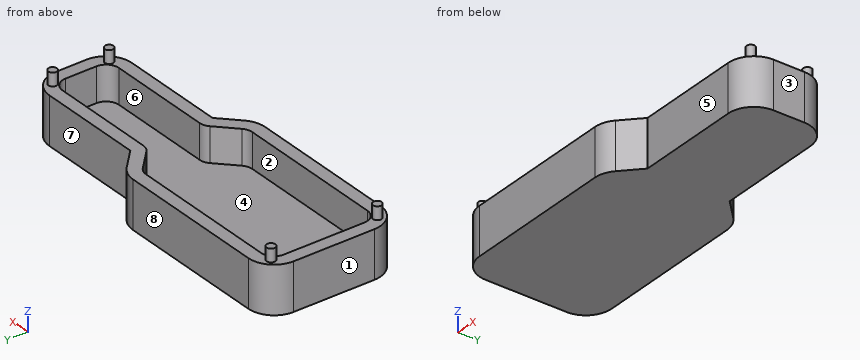
```python
from build123d import *

# Parameters (mm, degrees)
SKETCH3_R                = 1
BOSS_EXTRUDE2_DEPTH      = 8
BOSS_EXTRUDE2_DEPTH_BACK = 3
BOSS_EXTRUDE3_DEPTH      = 3
SKETCH7_R                = 1
BOSS_EXTRUDE4_DEPTH      = 3
BOSS_EXTRUDE4_DEPTH_BACK = 11


with BuildPart() as part:
    # Sketch3 → Boss-Extrude2 (new, two sides)
    with BuildSketch(Plane.XY) as boss_extrude2_sk:
        with BuildLine():
            Line((-69.81, 20.47), (-34.625063383, 20.47))
            ThreePointArc((-34.625063383, 20.47), (-32.391172348, 20.03863815), (-30.478486436, 18.806576947))
            Line((-30.478486436, 18.806576947), (-26.141909489, 14.66))
            Line((-26.141909489, 14.66), (-1.5, 14.66))
            ThreePointArc((-1.5, 14.66), (2.742640687, 12.902640687), (4.5, 8.66))
            Line((4.5, 8.66), (4.5, 1.5))
            ThreePointArc((4.5, 1.5), (2.742640687, -2.742640687), (-1.5, -4.5))
            Line((-1.5, -4.5), (-26.141909489, -4.5))
            Line((-26.141909489, -4.5), (-30.478486436, -8.646576947))
            ThreePointArc((-30.478486436, -8.646576947), (-32.391172348, -9.87863815), (-34.625063383, -10.31))
            Line((-34.625063383, -10.31), (-69.81, -10.31))
            ThreePointArc((-69.81, -10.31), (-74.052640687, -8.552640687), (-75.81, -4.31))
            Line((-75.81, -4.31), (-75.81, 14.47))
            ThreePointArc((-75.81, 14.47), (-74.052640687, 18.712640687), (-69.81, 20.47))
        make_face()
        with Locations((-72.81, 17.47)):
            Circle(SKETCH3_R, mode=Mode.SUBTRACT)
        with Locations((-72.81, -7.31)):
            Circle(SKETCH3_R, mode=Mode.SUBTRACT)
        with Locations((1.5, -1.5)):
            Circle(SKETCH3_R, mode=Mode.SUBTRACT)
        with Locations((1.5, 11.66)):
            Circle(SKETCH3_R, mode=Mode.SUBTRACT)
        with BuildLine():
            Line((-69.81, 17.47), (-34.625063383, 17.47))
            ThreePointArc((-34.625063383, 17.47), (-33.508117866, 17.254319075), (-32.55177491, 16.638288474))
            Line((-32.55177491, 16.638288474), (-28.215197962, 12.491711526))
            ThreePointArc((-28.215197962, 12.491711526), (-27.258855006, 11.875680925), (-26.141909489, 11.66))
            Line((-26.141909489, 11.66), (-1.5, 11.66))
            ThreePointArc((-1.5, 11.66), (0.621320344, 10.781320344), (1.5, 8.66))
            Line((1.5, 8.66), (1.5, 1.5))
            ThreePointArc((1.5, 1.5), (0.621320344, -0.621320344), (-1.5, -1.5))
            Line((-1.5, -1.5), (-26.141909489, -1.5))
            ThreePointArc((-26.141909489, -1.5), (-27.258855006, -1.715680925), (-28.215197962, -2.331711526))
            Line((-28.215197962, -2.331711526), (-32.55177491, -6.478288474))
            ThreePointArc((-32.55177491, -6.478288474), (-33.508117866, -7.094319075), (-34.625063383, -7.31))
            Line((-34.625063383, -7.31), (-69.81, -7.31))
            ThreePointArc((-69.81, -7.31), (-71.931320344, -6.431320344), (-72.81, -4.31))
            Line((-72.81, -4.31), (-72.81, 14.47))
            ThreePointArc((-72.81, 14.47), (-71.931320344, 16.591320344), (-69.81, 17.47))
        make_face(mode=Mode.SUBTRACT)
    extrude(amount=BOSS_EXTRUDE2_DEPTH)
    extrude(boss_extrude2_sk.sketch, amount=-BOSS_EXTRUDE2_DEPTH_BACK)

    # Sketch5 → Boss-Extrude3 (add)
    with BuildSketch(Plane(origin=(0, 0, -3), x_dir=(-1, 0, 0), z_dir=(0, 0, -1))):
        with BuildLine():
            Line((72.81, 14.47), (72.81, -4.31))
            ThreePointArc((72.81, -4.31), (71.931320344, -6.431320344), (69.81, -7.31))
            Line((69.81, -7.31), (34.625063383, -7.31))
            ThreePointArc((34.625063383, -7.31), (33.508117866, -7.094319075), (32.55177491, -6.478288474))
            Line((32.55177491, -6.478288474), (28.215197962, -2.331711526))
            ThreePointArc((28.215197962, -2.331711526), (27.258855006, -1.715680925), (26.141909489, -1.5))
            Line((26.141909489, -1.5), (1.5, -1.5))
            ThreePointArc((1.5, -1.5), (-0.621320344, -0.621320344), (-1.5, 1.5))
            Line((-1.5, 1.5), (-1.5, 8.66))
            ThreePointArc((-1.5, 8.66), (-0.621320344, 10.781320344), (1.5, 11.66))
            Line((1.5, 11.66), (26.141909489, 11.66))
            ThreePointArc((26.141909489, 11.66), (27.258855006, 11.875680925), (28.215197962, 12.491711526))
            Line((28.215197962, 12.491711526), (32.55177491, 16.638288474))
            ThreePointArc((32.55177491, 16.638288474), (33.508117866, 17.254319075), (34.625063383, 17.47))
            Line((34.625063383, 17.47), (69.81, 17.47))
            ThreePointArc((69.81, 17.47), (71.931320344, 16.591320344), (72.81, 14.47))
        make_face()
    extrude(amount=-BOSS_EXTRUDE3_DEPTH)

    # Sketch7 → Boss-Extrude4 (add, two sides)
    with BuildSketch(Plane.XY.offset(8)) as boss_extrude4_sk:
        with Locations((-72.81, 17.47)):
            Circle(SKETCH7_R)
        with Locations((1.5, -1.5)):
            Circle(SKETCH7_R)
        with Locations((1.5, 11.66)):
            Circle(SKETCH7_R)
        with Locations((-72.81, -7.31)):
            Circle(SKETCH7_R)
    extrude(amount=BOSS_EXTRUDE4_DEPTH)
    extrude(boss_extrude4_sk.sketch, amount=-BOSS_EXTRUDE4_DEPTH_BACK)


solid = part.part
```
Part model, mm, in its own coordinate system. Face numbers are marked on the shaded views. A direction names the side the tool comes from. Round coordinates to 2 decimals unless told otherwise and drop trailing zeros. Loops run counter-clockwise (first coordinate to the right, second up) from the corner with the lowest first, then second, coordinate; pieces in that order, holes last.
Item 1: Mould opens along X. For the marked faces 1, 2, 3 and 4 say: +X half, -X half, draft (parallel to the pull), parting line (faces both ways), or undercut.
Item 2: Drop flat-ended pins along their axis: P1, Ø6, axis at x = -30, z = 3, coming from the +Y side; P2, Ø3, axis at x = -19.5, y = 13, coming from the +Z side; P3, Ø6, axis at y = -4.5, z = 5, coming from the +X side; P4, Ø4, axis at x = -9.5, y = 17, coming from the -Z side. Give the stop position or say it passes through.
Item 3: Drill centre lines: line 1 (Y direction, x = -39, z = 1.5); line 2 (Y direction, x = -20.5, z = 3.25); line 3 (Y direction, x = -15, z = -1). Where is each one in solid material? Low to high.
Item 4: 3-axis set-ups, long thin cutter, end or side, ignore diameter. For the marked faces 5, 6, 7 and 8: which of +Z, -Z, +X, -X, +Y, -Y reach the whole face in a straight line?
Item 5: Cut at B-B, the plane x = -62. Give the cut face in (y, z).
A:
1. face 1: -X half
1. face 2: undercut
1. face 3: +X half
1. face 4: undercut
2. P1: stops at y = 20.25
2. P2: stops at z = 8
2. P3: stops at x = 3.7
2. P4: passes through
3. line 1: y = -10.31 to -7.31, 17.47 to 20.47
3. line 2: y = -4.5 to -1.5, 11.66 to 14.66
3. line 3: y = -4.5 to 14.66
4. face 5: +Z, -Z, +X, -Y
4. face 6: +Z
4. face 7: +Z, -Z, +X, +Y
4. face 8: +Z, -Z, +X, -X, +Y
5. outline: (-10.31, -3) - (20.47, -3) - (20.47, 8) - (17.47, 8) - (17.47, 0) - (-7.31, 0) - (-7.31, 8) - (-10.31, 8) - close
